Here's how the part is built. I have some questions about the finished solid (model axes, mm). Face numbers are marked on the shaded views. A direction names the side the tool comes from. Round coordinates to 2 decimals unless told otherwise and drop trailing zeros. Order: outer loops, then holes, each group sorted by start corner. A loop starts at its lowest first (then second) coordinate and runs counter-clockwise, first axis right, second up. Notation, with made-up numbers: (19, 65.5) -> (34, 65.5) arc R33 cw to (34, 99.5) -> close; hole circle Ø9 at (-32, 35.5). An arc over 180 degrees is marked (long way). Use a Markdown table: item, result. Add a question column.
(1) If I drill on probe 1 along Y at (x, z) = (8.5, 6.5); probe 2 along Y at (x, z) = (-10, -6.25); probe 3 along X at (y, z) = (10, 5.5), over which ranges is the centre line in solid material (lowest first)?
(2) Thinking about a two-plate mould opening in Y: for the marked faces 1, 2 and 3, which applies, pulls with the +Y half, pulls with the -Y half, needs draft (parallel to the pull), parting line crosses it, or undercut?
(3) I want a section at C-C, the plane z = 4.75. Please give me the cut outline in (x, y).
(4) I want a section at A-A, the plane x = 9.5. Please give me the cut outline in (y, z), then the cut area to 3 significant figures.
(5) I'm going to push flat-ended pins straight in: P1, Ø7.5, axis at x = 11, z = 7.5, coming from the -Y side; P2, Ø1.4, axis at y = 4, z = -4, coming from the -X side; P3, Ø3, axis at x = 13.19, y = 30.3, coming from the +Z side; P4, Ø5.5, axis at y = 15, z = 1, coming from the +X side. Where does each tip first touch, or does it pass through?
(6) I want a section at D-D, the plane x = -6. Please give me the cut outline in (y, z), then the cut area to 3 significant figures.
(7) On a 3-axis mill with a long thin cutter (end or side, diameter ignored), from which of +Z, -Z, +X, -X, +Y, -Y can I reach the whole of each face in a straight line? I mean the marked faces 4, 5 and 6. Say none if no direction works.
(8) I want a section at B-B, the plane y = 30.3. Please give me the cut outline in (x, z), then the cut area to 3 significant figures.
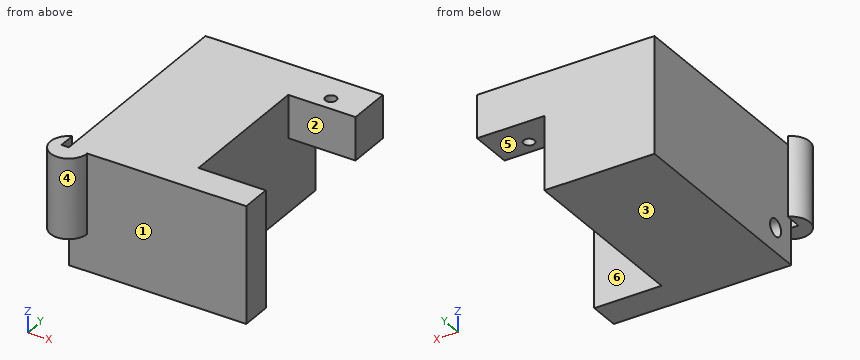
from build123d import *

# Parameters (mm, degrees)
SKETCH1_W           = 18
SKETCH1_H           = 19
BOSS_EXTRUDE1_DEPTH = 35
SKETCH2_W           = 19
SKETCH2_H           = 5
SKETCH2_H_2         = 7
BOSS_EXTRUDE2_DEPTH = 11
SKETCH3_W           = 12
SKETCH3_H           = 7
CUT_EXTRUDE1_DEPTH  = 11
SKETCH7_W           = 3
SKETCH7_H           = 19
SKETCH9_W           = 39
SKETCH9_H           = 6
CUT_EXTRUDE3_DEPTH  = 4
SKETCH10_W          = 6
SKETCH10_H          = 35
CUT_EXTRUDE4_DEPTH  = 4
SKETCH11_W          = 1.2
SKETCH11_H          = 19
CUT_EXTRUDE5_DEPTH  = 35
SKETCH12_R          = 1.4
CUT_EXTRUDE6_DEPTH  = 5
SKETCH13_R          = 0.9
CUT_EXTRUDE7_DEPTH  = 20


with BuildPart() as part:
    # Sketch1 → Boss-Extrude1 (new body)
    with BuildSketch(Plane(origin=(0, 0, 0), x_dir=(1, 0, 0), z_dir=(0, 1, 0))):
        with Locations((-1.30615381, -1.556170273)):
            Rectangle(SKETCH1_W, SKETCH1_H)
    extrude(amount=BOSS_EXTRUDE1_DEPTH)

    # Sketch2 → Boss-Extrude2 (add)
    with BuildSketch(Plane(origin=(7.69384619, 0, 0), x_dir=(0, 0, -1), z_dir=(1, 0, 0))):
        with Locations((-1.556170273, 2.5)):
            Rectangle(SKETCH2_W, SKETCH2_H)
        with Locations((-1.556170273, 31.5)):
            Rectangle(SKETCH2_W, SKETCH2_H_2)
    extrude(amount=BOSS_EXTRUDE2_DEPTH)

    # Sketch3 → Cut-Extrude1 (cut)
    with BuildSketch(Plane(origin=(18.69384619, 0, 0), x_dir=(0, 0, -1), z_dir=(1, 0, 0))):
        with Locations((1.943829727, 31.5)):
            Rectangle(SKETCH3_W, SKETCH3_H)
    extrude(amount=-CUT_EXTRUDE1_DEPTH, mode=Mode.SUBTRACT)

    # Sketch7 → Revolve2 (revolve)
    with BuildSketch(Plane.XZ):
        with Locations((-8.80615381, 1.556170273)):
            Rectangle(SKETCH7_W, SKETCH7_H)
    revolve(axis=Axis((-10.30615381, 0, -7.943829727), (0, 0, 1)))

    # Sketch9 → Cut-Extrude3 (cut, through all)
    with BuildSketch(Plane.XZ):
        with Locations((-0.80615381, -4.943829727)):
            Rectangle(SKETCH9_W, SKETCH9_H)
    extrude(amount=CUT_EXTRUDE3_DEPTH, mode=Mode.SUBTRACT)

    # Sketch10 → Cut-Extrude4 (cut, through all)
    with BuildSketch(Plane.ZY.offset(10.30615381)):
        with Locations((-4.943829727, 17.5)):
            Rectangle(SKETCH10_W, SKETCH10_H)
    extrude(amount=CUT_EXTRUDE4_DEPTH, mode=Mode.SUBTRACT)

    # Sketch11 → Cut-Extrude5 (cut)
    with BuildSketch(Plane(origin=(0, 35, 0), x_dir=(1, 0, 0), z_dir=(0, 1, 0))):
        with Locations((-10.90615381, -1.556170273)):
            Rectangle(SKETCH11_W, SKETCH11_H)
    extrude(amount=-CUT_EXTRUDE5_DEPTH, mode=Mode.SUBTRACT)

    # Sketch12 → Cut-Extrude6 (cut)
    with BuildSketch(Plane.ZY.offset(10.30615381)):
        with Locations((-3.943829727, 4)):
            Circle(SKETCH12_R)
    extrude(amount=-CUT_EXTRUDE6_DEPTH, mode=Mode.SUBTRACT)

    # Sketch13 → Cut-Extrude7 (cut, through all)
    with BuildSketch(Plane.XY.offset(11.056170273)):
        with Locations((13.19384619, 30.3)):
            Circle(SKETCH13_R)
    extrude(amount=-CUT_EXTRUDE7_DEPTH, mode=Mode.SUBTRACT)


solid = part.part
Taken from the geometry:
| question | item | result |
|---|---|---|
| 1 | probe 1 | y = 0 to 5, 28 to 35 |
| 1 | probe 2 | y = 0 to 35 |
| 1 | probe 3 | x = -10.31 to 7.69 |
| 2 | face 1 | pulls with the -Y half |
| 2 | face 2 | undercut |
| 2 | face 3 | needs draft |
| 3 | outline | (-11.51, 0) -> (-11.51, 2.75) arc R3 ccw (long way) to (-7.31, 0) -> (18.69, 0) -> (18.69, 5) -> (7.69, 5) -> (7.69, 28) -> (18.69, 28) -> (18.69, 35) -> (-10.31, 35) -> (-10.31, 0) -> close; hole circle Ø1.8 at (13.19, 30.3) |
| 4 | outline | (0, -7.94) -> (5, -7.94) -> (5, 11.06) -> (0, 11.06) -> close; (28, 4.06) -> (35, 4.06) -> (35, 11.06) -> (28, 11.06) -> close |
| 4 | area | 144 mm2 |
| 5 | P1 | stops at y = 0 |
| 5 | P2 | stops at x = -5.31 |
| 5 | P3 | stops at z = 11.06 |
| 5 | P4 | stops at x = 7.69 |
| 6 | outline | (0, -7.94) -> (35, -7.94) -> (35, 11.06) -> (0, 11.06) -> close; hole circle Ø2.8 at (4, -3.94) |
| 6 | area | 659 mm2 |
| 7 | face 4 | +Z, -Z |
| 7 | face 5 | -Z, +X, +Y |
| 7 | face 6 | +Z, -Z, +X |
| 8 | outline | (-10.31, -7.94) -> (7.69, -7.94) -> (7.69, 4.06) -> (12.29, 4.06) -> (12.29, 11.06) -> (-10.31, 11.06) -> close; (14.09, 4.06) -> (18.69, 4.06) -> (18.69, 11.06) -> (14.09, 11.06) -> close |
| 8 | area | 406 mm2 |
